CAD build for the part. Positions are in the model's coordinates, mm. A direction names the side the tool comes from. Give positions to 0.01 mm unless a question says otherwise; leave off trailing zeros. Write each loop counter-clockwise with the first axis right and the second up, starting at its lowest first coordinate (ties: lowest second). Pieces come first, ordered by that corner, then holes. Notation, with made-up numbers: (-34, 84) -> (0, 84) arc R13 ccw to (0, 92) -> close; hole circle Ø2 at (66.5, 35). An arc over 180 degrees is marked (long way). Answer in a Markdown table with one row per item. Add a question column.
```python
from build123d import *

# Parameters (mm, degrees)
SKETCH1_W           = 36
SKETCH1_H           = 36
SKETCH1_W_2         = 31.2
SKETCH1_H_2         = 31.2
BOSS_EXTRUDE1_DEPTH = 5.2
SKETCH2_W           = 36
SKETCH2_H           = 36
SKETCH2_W_2         = 21.6
SKETCH2_H_2         = 21.6
BOSS_EXTRUDE2_DEPTH = 1.2
SKETCH3_W           = 21.6
SKETCH3_H           = 21.6
SKETCH3_R           = 8.1
BOSS_EXTRUDE3_DEPTH = 1.2


with BuildPart() as part:
    # Sketch1 → Boss-Extrude1 (new body)
    with BuildSketch(Plane(origin=(0, 0, 0), x_dir=(1, 0, 0), z_dir=(0, 1, 0))):
        Rectangle(SKETCH1_W, SKETCH1_H)
        Rectangle(SKETCH1_W_2, SKETCH1_H_2, mode=Mode.SUBTRACT)
    extrude(amount=BOSS_EXTRUDE1_DEPTH)

    # Sketch2 → Boss-Extrude2 (add)
    with BuildSketch(Plane(origin=(0, 5.2, 0), x_dir=(1, 0, 0), z_dir=(0, 1, 0))):
        Rectangle(SKETCH2_W, SKETCH2_H)
        Rectangle(SKETCH2_W_2, SKETCH2_H_2, mode=Mode.SUBTRACT)
    extrude(amount=BOSS_EXTRUDE2_DEPTH)

    # Sketch3 → Boss-Extrude3 (add)
    with BuildSketch(Plane(origin=(0, 6.4, 0), x_dir=(1, 0, 0), z_dir=(0, 1, 0))):
        Rectangle(SKETCH3_W, SKETCH3_H)
        with Locations(Location((0, 0, 0), (0, 0, 270))):
            Circle(SKETCH3_R, mode=Mode.SUBTRACT)
    extrude(amount=-BOSS_EXTRUDE3_DEPTH)


solid = part.part
```
Item 1: Slice it at D-D, the plane x = -11. List the corners of the cut face in (y, z), then the cut area to 3 significant figures.
Item 2: Slice it at A-A, the plane z = 0. List the corners of the cut face in (x, y), then the cut area to 3 significant figures.
Item 3: Drop flat-ended pins along their axis: pin 1 Ø9.5 at (x, z) = (2.5, -5) entering from -Y; pin 2 Ø1.5 at (x, z) = (-5.5, 0) entering from -Y. Give the stop position or say it passes through.
Item 4: Mould opens along X. For faces 1 (the face through (7, 5.2, -7)), 2 (the face through (18, 3, 0)), 3 (the face through (-16, 0, 0)) say: released by +X, released by -X, zero draft, split by the parting line, or undercut.
Item 5: Slice it at B-B, the plane x = 0. List the corners of the cut face in (y, z), then the cut area to 3 significant figures.
Item 6: Probe L1, parallel to Z at x = -1, y = 1; L2, parallel to X at y = 6.15, z = 0. List the from-to ranges inside material, lowest first. Write a range as from..to.
Item 7: Slice it at C-C, the plane y = 3.5. List the corners of the cut face in (x, z).
Item 8: Which spindle directions (+Z, -Z, +X, -X, +Y, -Y) get a long thin tool onto all of the face, cutting with end or side? Do faces 4 (the face through (0, 3, 18)), 5 (the face through (-15.6, 3, 0)). Say none if no direction does.
Answer key:
| question | item | result |
|---|---|---|
| 1 | outline | (0, -18) -> (6.4, -18) -> (6.4, 18) -> (0, 18) -> (0, 15.6) -> (5.2, 15.6) -> (5.2, -15.6) -> (0, -15.6) -> close |
| 1 | area | 68.2 mm² |
| 2 | outline | (-18, 0) -> (-15.6, 0) -> (-15.6, 5.2) -> (-8.1, 5.2) -> (-8.1, 6.4) -> (-18, 6.4) -> close; (8.1, 5.2) -> (15.6, 5.2) -> (15.6, 0) -> (18, 0) -> (18, 6.4) -> (8.1, 6.4) -> close |
| 2 | area | 48.7 mm² |
| 3 | pin 1 | stops at y = 5.2 |
| 3 | pin 2 | passes through |
| 4 | face 1 | undercut |
| 4 | face 2 | released by +X |
| 4 | face 3 | zero draft |
| 5 | outline | (0, -18) -> (6.4, -18) -> (6.4, -8.1) -> (5.2, -8.1) -> (5.2, -15.6) -> (0, -15.6) -> close; (0, 15.6) -> (5.2, 15.6) -> (5.2, 8.1) -> (6.4, 8.1) -> (6.4, 18) -> (0, 18) -> close |
| 5 | area | 48.7 mm² |
| 6 | L1 | z = -18..-15.6, 15.6..18 |
| 6 | L2 | x = -18..-8.1, 8.1..18 |
| 7 | outline | (-18, -18) -> (18, -18) -> (18, 18) -> (-18, 18) -> close; hole (-15.6, -15.6) -> (15.6, -15.6) -> (15.6, 15.6) -> (-15.6, 15.6) -> close |
| 8 | face 4 | +Z, +X, -X, +Y, -Y |
| 8 | face 5 | -Y |
